Source: three-view drawing plus pictorial views. Frame: mm from the lowest corner of the part. Give positions to 0.01 mm unless a question says otherwise; leave off trailing zeros. Order: outer loops, then holes, each group sorted by start corner. A loop starts at its lowest first (then second) coordinate and runs counter-clockwise, first axis right, second up. Notation, with made-up numbers: (79.5, -31.75) - (94.5, -31.75) arc R18 ccw to (94.5, 1.25) - close; hole circle Ø4 at (-5, 68). An arc over 180 degrees is marked (long way). Answer in a Markdown table with one row per item. Add a question column.
1. Section query B-B on x = 13.97. Return loops of the section in (y, z) (1 decimal), and give its area (3 significant figures).
2. Mould query, pull axis X, two halves, no side actions, for the marked faces 1, 2, 3 and 4. Classes: released by +X, released by -X, zero draft, split by the parting line, or undercut.
3. Section query D-D on y = 15. Return loops of the section in (x, z) (3 decimals).
4. Contact query for flat-ended pins moving along their axis: pin 1 (1.6 mm diameter, centred on y = 27.5, z = 1, fed in from -X); pin 2 (1.6 mm diameter, centred on y = 2.5, z = 1, fed in from -X); pin 3 (1 mm diameter, centred on y = 28, z = 1, fed in from +X). Output: stop coordinate, or through.
5. Ray query, line 1 (Y direction, x = 13.97, z = 2.45); line 2 (X direction, y = 2.5, z = 2.2); line 3 (X direction, y = 20, z = 0.6). Return the intervals inside material, ascending. Write a range as [from, to].
6. Section query C-C on y = 28. Return loops of the section in (x, z) (3 decimals), and give its area (3 significant figures).
7. Section query A-A on z = 1.95. Return loops of the section in (x, y) (1 decimal), and give its area (3 significant figures).
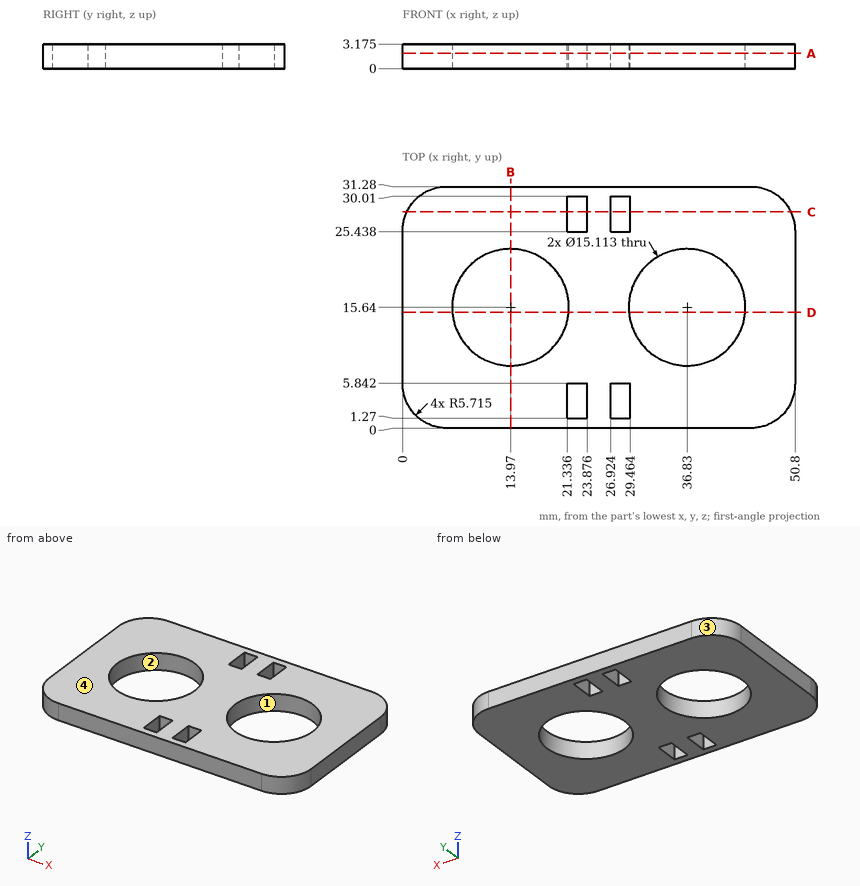
Answer:
| question | item | result |
|---|---|---|
| 1 | outline | (0, 0) - (8.1, 0) - (8.1, 3.2) - (0, 3.2) - close; (23.2, 0) - (31.3, 0) - (31.3, 3.2) - (23.2, 3.2) - close |
| 1 | area | 51.3 mm² |
| 2 | face 1 | undercut |
| 2 | face 2 | undercut |
| 2 | face 3 | released by -X |
| 2 | face 4 | zero draft |
| 3 | outline | (0, 0) - (6.441, 0) - (6.441, 3.175) - (0, 3.175) - close; (21.499, 0) - (29.301, 0) - (29.301, 3.175) - (21.499, 3.175) - close; (44.359, 0) - (50.8, 0) - (50.8, 3.175) - (44.359, 3.175) - close |
| 4 | pin 1 | stops at x = 0.11 |
| 4 | pin 2 | stops at x = 0.54 |
| 4 | pin 3 | stops at x = 50.46 |
| 5 | line 1 | y = [0, 8.08], [23.2, 31.28] |
| 5 | line 2 | x = [0.99, 21.34], [23.88, 26.92], [29.46, 49.81] |
| 5 | line 3 | x = [0, 7.8], [20.14, 30.66], [43, 50.8] |
| 6 | outline | (0.545, 0) - (21.336, 0) - (21.336, 3.175) - (0.545, 3.175) - close; (23.876, 0) - (26.924, 0) - (26.924, 3.175) - (23.876, 3.175) - close; (29.464, 0) - (50.255, 0) - (50.255, 3.175) - (29.464, 3.175) - close |
| 6 | area | 142 mm² |
| 7 | outline | (0, 5.7) arc R5.7 ccw to (5.7, 0) - (45.1, 0) arc R5.7 ccw to (50.8, 5.7) - (50.8, 25.6) arc R5.7 ccw to (45.1, 31.3) - (5.7, 31.3) arc R5.7 ccw to (0, 25.6) - close; hole circle Ø15.1 at (14, 15.6); hole (21.3, 1.3) - (23.9, 1.3) - (23.9, 5.8) - (21.3, 5.8) - close; hole (21.3, 25.4) - (23.9, 25.4) - (23.9, 30) - (21.3, 30) - close; hole (26.9, 1.3) - (29.5, 1.3) - (29.5, 5.8) - (26.9, 5.8) - close; hole (26.9, 25.4) - (29.5, 25.4) - (29.5, 30) - (26.9, 30) - close; hole circle Ø15.1 at (36.8, 15.6) |
| 7 | area | 1,160 mm² |
